```python
from build123d import *

# Parameters (mm, degrees)
SKICA1_W                 = 72.5
SKICA1_H                 = 27.5
P_IDAT_VYSUNUT_M1_DEPTH  = 2
SKICA2_W                 = 68.5
SKICA2_H                 = 23.5
P_IDAT_VYSUNUT_M2_DEPTH  = 1.5
SKICA3_W                 = 14.5
SKICA3_H                 = 16
SKICA3_W_2               = 5.3
SKICA3_H_2               = 2.2
ODEBRAT_VYSUNUT_M1_DEPTH = 39.927817817


with BuildPart() as part:
    # Skica1 → Přidat vysunutím1 (new body)
    with BuildSketch(Plane.XY):
        Rectangle(SKICA1_W, SKICA1_H)
    extrude(amount=P_IDAT_VYSUNUT_M1_DEPTH)

    # Skica2 → Přidat vysunutím2 (add)
    with BuildSketch(Plane.XY.offset(2)):
        Rectangle(SKICA2_W, SKICA2_H)
    extrude(amount=P_IDAT_VYSUNUT_M2_DEPTH)

    # Skica3 → Odebrat vysunutím1 (cut, through all)
    with BuildSketch(Plane.XY.offset(3.5)):
        with Locations((16.65, 0.25)):
            Rectangle(SKICA3_W, SKICA3_H)
        with Locations((-3.35, 0.25)):
            Rectangle(SKICA3_W, SKICA3_H)
        with Locations((-23.85, 0.25)):
            Rectangle(SKICA3_W, SKICA3_H)
        with Locations((30.4, -6.65)):
            Rectangle(SKICA3_W_2, SKICA3_H_2)
    extrude(amount=-ODEBRAT_VYSUNUT_M1_DEPTH, mode=Mode.SUBTRACT)


solid = part.part
```
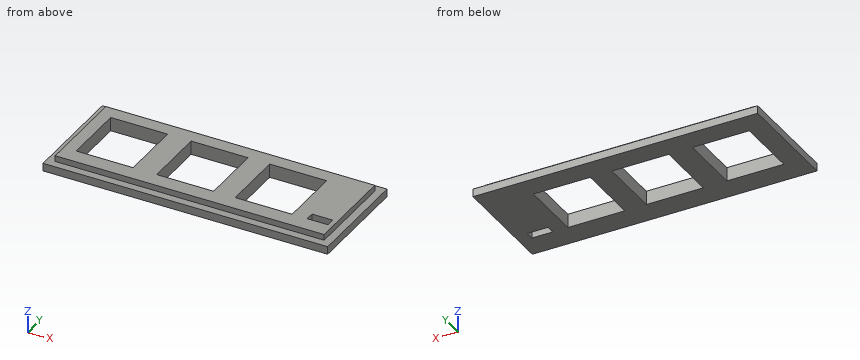
The listing builds one solid part. Answer for the finished solid, in the listing's coordinates (mm). Round coordinates to 2 decimals unless told otherwise and drop trailing zeros. Loops run counter-clockwise (first coordinate to the right, second up) from the corner with the lowest first, then second, coordinate; pieces in that order, holes last. Notation, with made-up numbers: (-24, 82) -> (13, 82) arc R28 cw to (13, 110) -> close; hole circle Ø9 at (23, 19.5). An arc over 180 degrees is marked (long way). Use one line per item in the form item = value.
1. Find the intervals of material crossed by probe 1 along X at (y, z) = (-3, 2.3); probe 2 along X at (y, z) = (3, 1.2); probe 3 along Y at (x, z) = (22, 1.6), in increasing order. Write a range as [from, to].
Answer key:
probe_1 = [-34.25, -31.1], [-16.6, -10.6], [3.9, 9.4], [23.9, 34.25]
probe_2 = [-36.25, -31.1], [-16.6, -10.6], [3.9, 9.4], [23.9, 36.25]
probe_3 = [-13.75, -7.75], [8.25, 13.75]
2. The part is cut by section A-A on x = -3.5. Determine the outline of the cut face in (y, z), and give its area (4 significant figures).
Answer key:
outline = (-13.75, 0) -> (-7.75, 0) -> (-7.75, 3.5) -> (-11.75, 3.5) -> (-11.75, 2) -> (-13.75, 2) -> close; (8.25, 0) -> (13.75, 0) -> (13.75, 2) -> (11.75, 2) -> (11.75, 3.5) -> (8.25, 3.5) -> close
area = 34.25 mm²
3. The part is cut by section D-D on y = -2.5. Determine the outline of the cut face in (x, z).
Answer key:
outline = (-36.25, 0) -> (-31.1, 0) -> (-31.1, 3.5) -> (-34.25, 3.5) -> (-34.25, 2) -> (-36.25, 2) -> close; (-16.6, 0) -> (-10.6, 0) -> (-10.6, 3.5) -> (-16.6, 3.5) -> close; (3.9, 0) -> (9.4, 0) -> (9.4, 3.5) -> (3.9, 3.5) -> close; (23.9, 0) -> (36.25, 0) -> (36.25, 2) -> (34.25, 2) -> (34.25, 3.5) -> (23.9, 3.5) -> close
4. Flat-ended cylindrical pins translate along their axes: pin 1 Ø0.8 at (x, z) = (-6, 2.5) entering from -Y; pin 2 Ø1.6 at (x, z) = (7.5, 3) entering from +Y. Find the tip coordinate at first contact, or state that the pin passes through.
Answer key:
pin_1 = -11.75
pin_2 = 11.75
5. The part is cut by section C-C on y = -6.5. Determine the outline of the cut face in (x, z).
Answer key:
outline = (-36.25, 0) -> (-31.1, 0) -> (-31.1, 3.5) -> (-34.25, 3.5) -> (-34.25, 2) -> (-36.25, 2) -> close; (-16.6, 0) -> (-10.6, 0) -> (-10.6, 3.5) -> (-16.6, 3.5) -> close; (3.9, 0) -> (9.4, 0) -> (9.4, 3.5) -> (3.9, 3.5) -> close; (23.9, 0) -> (27.75, 0) -> (27.75, 3.5) -> (23.9, 3.5) -> close; (33.05, 0) -> (36.25, 0) -> (36.25, 2) -> (34.25, 2) -> (34.25, 3.5) -> (33.05, 3.5) -> close
6. The part is cut by section B-B on z = 2.75. Determine the outline of the cut face in (x, y), and give its area (3 significant figures).
Answer key:
outline = (-34.25, -11.75) -> (34.25, -11.75) -> (34.25, 11.75) -> (-34.25, 11.75) -> close; hole (-31.1, -7.75) -> (-16.6, -7.75) -> (-16.6, 8.25) -> (-31.1, 8.25) -> close; hole (-10.6, -7.75) -> (3.9, -7.75) -> (3.9, 8.25) -> (-10.6, 8.25) -> close; hole (9.4, -7.75) -> (23.9, -7.75) -> (23.9, 8.25) -> (9.4, 8.25) -> close; hole (27.75, -7.75) -> (33.05, -7.75) -> (33.05, -5.55) -> (27.75, -5.55) -> close
area = 902 mm²
